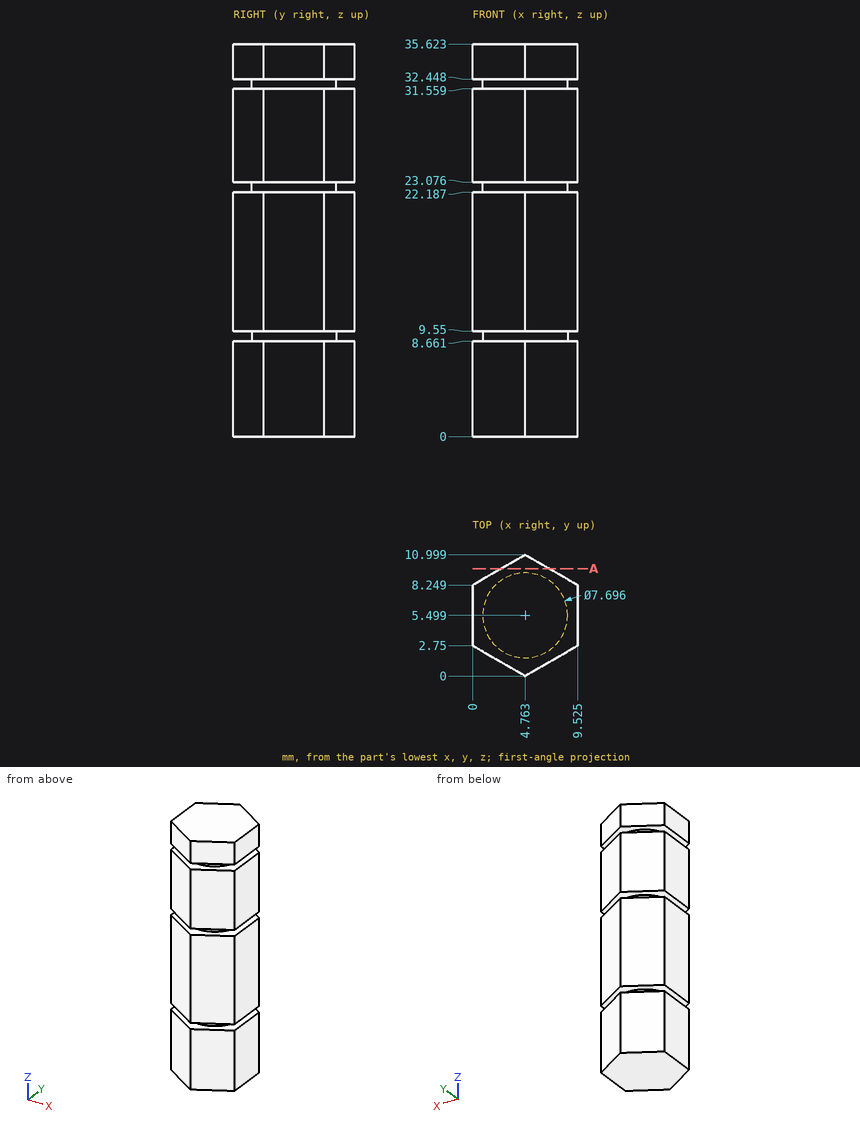
Here's the drawing with two shaded views (mm, measured from the low corner). I have some questions. Coordinates: 2 decimals unless noted, no trailing zeros. Answer as CSV lines item,"result".
Item 1: For pin 1 (3 mm diameter, centred on x = 3.5, z = 17, fed in from +Y); pin 2 (4 mm diameter, centred on x = 2, z = 12, fed in from +Y); pin 3 (1 mm diameter, centred on x = 3.5, z = 4, fed in from -Y), each with a flat end and sliding along its axis, tell me the tip position at first contact or that it passes through.
Results found:
pin 1,"y = 11"
pin 2,"y = 10.56"
pin 3,"y = 0.44"
Item 2: Imagine slicing it at A-A on y = 9.75. Give the number of separate pieces and of enclosed holes in the cut face.
Results found:
separate pieces,"4"
enclosed holes,"0"
Item 3: If I drill on line 1 (Y direction, x = 7.75, z = 17.5) (1 decimal); line 2 (X direction, y = 2, z = 28.5) (1 decimal); line 3 (Y direction, x = 1.25, z = 21.5), over which ranges is the centre line in solid material (lowest first)?
Results found:
line 1,"1.7 to 9.3"
line 2,"1.3 to 8.2"
line 3,"2.03 to 8.97"
